```python
from build123d import *

# Parameters (mm, degrees)
BOSS_EXTRUDE1_DEPTH = 4
BOSS_EXTRUDE1_TAPER = 10
CUT_EXTRUDE1_START  = 4
SKETCH1_3_R         = 1.1
CUT_EXTRUDE1_DEPTH  = 4
CUT_EXTRUDE2_START  = 4
SKETCH1_4_R         = 8.4
SKETCH1_4_R_2       = 1.1
CUT_EXTRUDE2_DEPTH  = 3


with BuildPart() as part:
    # Sketch1 → Boss-Extrude1 (new body)
    with BuildSketch(Plane(origin=(0, 0, 0), x_dir=(1, 0, 0), z_dir=(0, 1, 0))):
        with BuildLine():
            ThreePointArc((-19.8, 11.4), (-25.5, 9.872689603), (-29.672689603, 5.7))
            Line((-29.672689603, 5.7), (-39.572689603, -11.447302995))
            ThreePointArc((-39.572689603, -11.447302995), (-39.572689603, -22.847302995), (-29.7, -28.547302995))
            Line((-29.7, -28.547302995), (-9.9, -28.547302995))
            ThreePointArc((-9.9, -28.547302995), (-4.2, -27.019992598), (-0.027310397, -22.847302995))
            Line((-0.027310397, -22.847302995), (9.872689603, -5.7))
            ThreePointArc((9.872689603, -5.7), (9.872689603, 5.7), (0, 11.4))
            Line((0, 11.4), (-19.8, 11.4))
        make_face()
    extrude(amount=BOSS_EXTRUDE1_DEPTH, taper=BOSS_EXTRUDE1_TAPER)

    # Sketch1<3> → Cut-Extrude1 (cut)
    with BuildSketch(Plane(origin=(0, 0, 0), x_dir=(1, 0, 0), z_dir=(0, 1, 0)).offset(CUT_EXTRUDE1_START)):
        with Locations(Location((-9.9, -17.147302995, 0), (0, 0, 270))):
            Circle(SKETCH1_3_R)
        with Locations(Location((0, 0, 0), (0, 0, 270))):
            Circle(SKETCH1_3_R)
        with Locations(Location((-29.7, -17.147302995, 0), (0, 0, 270))):
            Circle(SKETCH1_3_R)
        with Locations(Location((-19.8, 0, 0), (0, 0, 270))):
            Circle(SKETCH1_3_R)
    extrude(amount=-CUT_EXTRUDE1_DEPTH, mode=Mode.SUBTRACT)

    # Sketch1<4> → Cut-Extrude2 (cut)
    # profile 1 of 4: a face of its own
    with BuildSketch(Plane(origin=(0, 0, 0), x_dir=(1, 0, 0), z_dir=(0, 1, 0)).offset(CUT_EXTRUDE2_START)):
        with Locations(Location((-19.8, 0, 0), (0, 0, 270))):
            Circle(SKETCH1_4_R)
        with Locations(Location((-19.8, 0, 0), (0, 0, 270))):
            Circle(SKETCH1_4_R_2, mode=Mode.SUBTRACT)
    # profile 2 of 4: a face of its own
    with BuildSketch(Plane(origin=(0, 0, 0), x_dir=(1, 0, 0), z_dir=(0, 1, 0)).offset(CUT_EXTRUDE2_START)):
        with Locations(Location((-9.9, -17.147302995, 0), (0, 0, 270))):
            Circle(SKETCH1_4_R)
        with Locations(Location((-9.9, -17.147302995, 0), (0, 0, 270))):
            Circle(SKETCH1_4_R_2, mode=Mode.SUBTRACT)
    # profile 3 of 4: a face of its own
    with BuildSketch(Plane(origin=(0, 0, 0), x_dir=(1, 0, 0), z_dir=(0, 1, 0)).offset(CUT_EXTRUDE2_START)):
        with Locations(Location((0, 0, 0), (0, 0, 270))):
            Circle(SKETCH1_4_R)
        with Locations(Location((0, 0, 0), (0, 0, 270))):
            Circle(SKETCH1_4_R_2, mode=Mode.SUBTRACT)
    # profile 4 of 4: a face of its own
    with BuildSketch(Plane(origin=(0, 0, 0), x_dir=(1, 0, 0), z_dir=(0, 1, 0)).offset(CUT_EXTRUDE2_START)):
        with Locations(Location((-29.7, -17.147302995, 0), (0, 0, 270))):
            Circle(SKETCH1_4_R)
        with Locations(Location((-29.7, -17.147302995, 0), (0, 0, 270))):
            Circle(SKETCH1_4_R_2, mode=Mode.SUBTRACT)
    extrude(amount=-CUT_EXTRUDE2_DEPTH, mode=Mode.SUBTRACT)


solid = part.part
```
Build history of the part. All positions in model axes, mm. A direction names the side the tool comes from. Give positions to 0.01 mm unless a question says otherwise; leave off trailing zeros. Return JSON: item names as keys, results as strings.
Q1. Wall check: probe 1 along X at (y, z) = (0.3, 0); probe 2 along X at (y, z) = (2.6, 15.5); probe 3 along Y at (x, z) = (-29, 25). Give the ranges that are in metal, low to high. Write a range as from..to.
Answer list:
{"probe 1": "x = -32.9..-20.9, -18.7..-1.1, 1.1..11.35", "probe 2": "x = -40.52..-37.94, -21.46..-18.14, -1.66..3.69", "probe 3": "y = 0..1"}
Q2. Band-saw the part on A-A (y = 2.55). Count the separate pieces of the cut face and the enclosed holes in it, then the cut area to 3 significant figures.
Answer list:
{"separate pieces": "1", "enclosed holes": "4", "area": "697 mm^2"}
Q3. Two-plate mould, pull along Z, no slides. Class faces 1 (the face through (-27.25, 2.52, 3.88)), 2 (the face through (-15, 0, 9)): pulls with the +Z half, pulls with the -Z half, needs draft (parallel to the pull), parting line crosses it, or undercut.
Answer list:
{"face 1": "undercut", "face 2": "needs draft"}
Q4. Flat gauge pins, fed straight in: pin 1 (3 mm diameter, centred on x = -9.9, z = 17.15, fed in from +Y); pin 2 (1 mm diameter, centred on y = 3, z = 20, fed in from +X); pin 3 (2 mm diameter, centred on y = 2.5, z = 6, fed in from -X). Where does each tip first touch, or does it go through?
Answer list:
{"pin 1": "stops at y = 1", "pin 2": "stops at x = 1.31", "pin 3": "stops at x = -36.53"}
Q5. 3-axis set-ups, long thin cutter, end or side, ignore diameter. For faces 3 (the face through (-9.531, 2.521, 8.755)), 4 (the face through (-29, 0.5, 16.3)): which of +Z, -Z, +X, -X, +Y, -Y reach the whole face in a straight line?
Answer list:
{"face 3": "+Y", "face 4": "+Y, -Y"}
